from build123d import *

# Parameters (mm, degrees)
ESQUISSE1_R                            = 45
BOSS_EXTRU_1_DEPTH                     = 1150
ESQUISSE2_R                            = 42
ENL_V_MAT_EXTRU_1_DEPTH                = 1150
ESQUISSE3_W                            = 10
ESQUISSE3_H                            = 3
ENL_V_MAT_EXTRU_2_DEPTH                = 200
R_P_TITION_CIRCULAIRE1_COUNT           = 4
ESQUISSE5_W                            = 2.75
ESQUISSE5_H                            = 90
D_GAGEMENT_M51_AT_2_COUNT              = 2
D_GAGEMENT_M51_AT_2_PITCH              = 214.601725843
R_P_TITION_CIRCULAIRE2_COUNT           = 2
R_P_TITION_CIRCULAIRE2_ANGLE           = 90
R_P_TITION_CIRCULAIRE2_COPY_1_SKETCH_W = 2.75
R_P_TITION_CIRCULAIRE2_COPY_1_SKETCH_H = 90


with BuildPart() as part:
    # Esquisse1 → Boss.-Extru.1 (new body)
    with BuildSketch(Plane.XY):
        Circle(ESQUISSE1_R)
    extrude(amount=BOSS_EXTRU_1_DEPTH)

    # Esquisse2 → Enlèv. mat.-Extru.1 (cut)
    with BuildSketch(Plane(origin=(0, 0, 0), x_dir=(-1, 0, 0), z_dir=(0, 0, -1))):
        Circle(ESQUISSE2_R)
    extrude(amount=-ENL_V_MAT_EXTRU_1_DEPTH, mode=Mode.SUBTRACT)

    # Esquisse3 → Enlèv. mat.-Extru.2 (cut)
    with BuildSketch(Plane.XY):
        with Locations((-45, 0)):
            Rectangle(ESQUISSE3_W, ESQUISSE3_H)
    enl_v_mat_extru_2 = extrude(amount=ENL_V_MAT_EXTRU_2_DEPTH, mode=Mode.SUBTRACT)

    # Répétition circulaire1: Enlèv. mat.-Extru.2 ×4 about axis
    r_p_tition_circulaire1_axis = Axis((0, 0, 0), (0, 0, 1))
    for i in range(1, R_P_TITION_CIRCULAIRE1_COUNT):
        add(enl_v_mat_extru_2.rotate(r_p_tition_circulaire1_axis, i * 360 / R_P_TITION_CIRCULAIRE1_COUNT), mode=Mode.SUBTRACT)

    # Esquisse5 → Dégagement M51 (revolve, cut)
    with BuildSketch(Plane(origin=(-45, 0, 206), x_dir=(0, 0, 1), z_dir=(0, 1, 0))):
        with Locations((1.375, 45)):
            Rectangle(ESQUISSE5_W, ESQUISSE5_H)
    d_gagement_m51 = revolve(axis=Axis((-51.35, 0, 206), (1, 0, 0)), mode=Mode.SUBTRACT)

    # Dégagement M51 at 2: Dégagement M51 ×2
    with Locations(*[Vector(0, -0.280281939, -0.959917723) * (i * D_GAGEMENT_M51_AT_2_PITCH) for i in range(1, D_GAGEMENT_M51_AT_2_COUNT)]):
        add(d_gagement_m51, mode=Mode.SUBTRACT)

    # Répétition circulaire2: Dégagement M51 ×2 about axis
    r_p_tition_circulaire2_axis = Axis((0, 0, 0), (0, 0, 1))
    for i in range(1, R_P_TITION_CIRCULAIRE2_COUNT):
        add(d_gagement_m51.rotate(r_p_tition_circulaire2_axis, i * R_P_TITION_CIRCULAIRE2_ANGLE / (R_P_TITION_CIRCULAIRE2_COUNT - 1)), mode=Mode.SUBTRACT)

    # Répétition circulaire2 copy 1 sketch → Répétition circulaire2 copy 1 (revolve, cut)
    with BuildSketch(Plane(origin=(60.14898781, -45, 0), x_dir=(0, 0, 1), z_dir=(-1, 0, 0))):
        with Locations((1.375, 45)):
            Rectangle(R_P_TITION_CIRCULAIRE2_COPY_1_SKETCH_W, R_P_TITION_CIRCULAIRE2_COPY_1_SKETCH_H)
    revolve(axis=Axis((60.14898781, -51.35, 0), (0, 1, 0)), mode=Mode.SUBTRACT)


solid = part.part
For this review, take the finished solid that the model builds, in its own axes (mm). Give positions to 0.01 mm unless a question says otherwise; leave off trailing zeros. Write each loop counter-clockwise with the first axis right and the second up, starting at its lowest first coordinate (ties: lowest second). Pieces come first, ordered by that corner, then holes. Notation, with made-up numbers: (49, 14) -> (104, 14) arc R13 cw to (104, 34) -> close; hole circle Ø5 at (10.25, 61.25). An arc over 180 degrees is marked (long way). Use CSV: the item, a comma, the result in double quotes.
Q1. Take a section at B-B, the plane x = 15.5. Write out the cut boundary in (y, z), then the cut area to 3 significant figures.
Conclusion:
outline,"(-42.25, 0) -> (-39.04, 0) -> (-39.04, 1150) -> (-42.25, 1150) -> close; (39.04, 0) -> (42.25, 0) -> (42.25, 1150) -> (39.04, 1150) -> close"
area,"7,390 mm2"
Q2. Take a section at C-C, the plane y = 27. Write out the cut boundary in (x, z), then the cut area to 3 significant figures.
Conclusion:
outline,"(-36, 0) -> (-32.17, 0) -> (-32.17, 1150) -> (-36, 1150) -> close; (32.17, 0) -> (36, 0) -> (36, 1150) -> (32.17, 1150) -> close"
area,"8,810 mm2"
Q3. Mouldability with a two-part tool opening along X and no side actions: class faces 1 (the face through (20.765, -39.923, 566.95)), 2 (the face through (-30, 30, 0)), 3 (the face through (-40.06, 12.62, 566.95)) as pulls with the +X half, pulls with the -X half, needs draft (parallel to the pull), parting line crosses it, or undercut.
Conclusion:
face 1,"parting line crosses it"
face 2,"needs draft"
face 3,"undercut"
Q4. For P1, Ø1.5, axis at x = -8.5, z = 476, coming from the -Y side; P2, Ø1, axis at x = -5.5, z = 898, coming from the +Y side; P3, Ø3, axis at y = -5.5, z = 260.5, coming from the -X side; P4, Ø5, axis at x = 0, z = 206, coming from the +Y side, all flat-tipped, find the tip position at first contact; note any pin that passes through.
Conclusion:
P1,"y = -44.33"
P2,"y = 44.72"
P3,"x = -44.82"
P4,"through"
Q5. Take a section at A-A, the plane z = 146.5. Write out the cut boundary in (x, y) (3 decimals), then the cut area to 3 significant figures.
Conclusion:
outline,"(-44.975, -1.5) arc R45 ccw to (-1.5, -44.975) -> (-1.5, -41.973) arc R42 cw to (-41.973, -1.5) -> close; (-44.975, 1.5) -> (-41.973, 1.5) arc R42 cw to (-1.5, 41.973) -> (-1.5, 44.975) arc R45 ccw to start; (1.5, -44.975) arc R45 ccw to (44.975, -1.5) -> (41.973, -1.5) arc R42 cw to (1.5, -41.973) -> close; (1.5, 41.973) arc R42 cw to (41.973, 1.5) -> (44.975, 1.5) arc R45 ccw to (1.5, 44.975) -> close"
area,"784 mm2"
Q6. To check wall thickness, follow probe 1 along X at (y, z) = (0, 659); probe 2 along Z at (x, y) = (-42.6, 0); probe 3 along Y at (x, z) = (-33.5, 116). State the ranges of each line that lie inside material, in increasing order. Write a range as [from, to].
Conclusion:
probe 1,"[-45, -42], [42, 45]"
probe 2,"[200, 203.25], [208.75, 1150]"
probe 3,"[-30.05, -25.33], [25.33, 30.05]"
